Autodesk Inventor part; units mm, degrees
ref_plane "YZ Plane" through (0, 0, 0) normal (1, 0, 0) x (0, 1, 0)
ref_plane "XZ Plane" through (0, 0, 0) normal (0, 1, 0) x (-1, 0, 0)
ref_plane "XY Plane" through (0, 0, 0) normal (0, 0, 1) x (1, 0, 0)
sketch "Boceto1" plane through (0, 0, 0) normal (0, 1, 0) x (-1, 0, 0)
  circle A0 centre (0, 0) radius 10
  circle A1 centre (0, 0) radius 3.5
  dimension "d0" = 20
  dimension "d1" = 7
extrude "Extrusión1" add sketch "Boceto1" along normal blind 4
sketch "Boceto2" plane through (0, 4, 0) normal (0, 1, 0) x (1, 0, 0)
  circle A0 centre (0, 0) radius 8
  circle A1 centre (0, 0) radius 3.5
  circle A2 centre (0, 0) radius 10
  dimension "d4" = 16
extrude "Extrusión2" cut sketch "Boceto2" against normal blind 3 contours A2
sketch "Boceto3" plane through (0, 4, 0) normal (0, 1, 0) x (1, 0, 0)
  circle A0 centre (0, 0) radius 8
  circle A1 centre (0, 0) radius 3.5
  circle A2 centre (0, 0) radius 10
  dimension "d7" = 16
extrude "Extrusión3" add sketch "Boceto3" against normal blind 1 contours A2
fillet "Empalme1" radius 0.5 4 edges at (-8, 1, 0) (-8, 3, 0) (-10, 3, 0) (10, 1, 0)
properties part number "servo pulley"
Read the model definition and answer for the solid it produces. Units are mm, in the model's axes. A direction names the side the tool comes from. Coordinates: 2 decimals unless noted, no trailing zeros. Loops run counter-clockwise (first coordinate to the right, second up) from the corner with the lowest first, then second, coordinate; pieces in that order, holes last.
Q1. Which of the six approach directions +Z, -Z, +X, -X, +Y, -Y give full straight-line access (tool end or side, diameter ignored) to faces 4 (the face through (-4, 0, 0)), 5 (the face through (-2.2, 3, 8.4))?
Q2. Consider probe 1 along Y at (x, z) = (6.25, 7.25); probe 2 along Z at (x, y) = (0, 1.85); probe 3 along Z at (x, y) = (-2, 0.2). Determine where each line is inside the solid, lowest interval first.
Q3. The mould has two halves that part along X. Classify faces 1 (the face through (2.17, 0.25, 9.76)), 2 (the face through (-3.233, 1.972, 1.341)), 3 (the face through (-2.2, 1, 8.4)): +X half, -X half, draft (parallel to the pull), parting line (faces both ways), or undercut.
Q4. The part is cut by section A-A on x = 0. Write down the section's boundary in (y, z).
Q5. The part is cut by section B-B on z = 0. Write down the section's boundary in (x, y), and give its area (3 significant figures).
Results below:
1. face 4: +Z, -Z, +X, -X, -Y
1. face 5: none
2. probe 1: y = 0 to 0.99, 3.01 to 4
2. probe 2: z = -8 to -3.5, 3.5 to 8
2. probe 3: z = -9.8 to -2.87, 2.87 to 9.8
3. face 1: parting line
3. face 2: undercut
3. face 3: draft
4. outline: (0, -10) - (0.5, -10) arc R0.5 ccw to (1, -9.5) - (1, -8.5) arc R0.5 cw to (1.5, -8) - (2.5, -8) arc R0.5 cw to (3, -8.5) - (3, -9.5) arc R0.5 ccw to (3.5, -10) - (4, -10) - (4, -3.5) - (0, -3.5) - close; (0, 3.5) - (4, 3.5) - (4, 10) - (3.5, 10) arc R0.5 ccw to (3, 9.5) - (3, 8.5) arc R0.5 cw to (2.5, 8) - (1.5, 8) arc R0.5 cw to (1, 8.5) - (1, 9.5) arc R0.5 ccw to (0.5, 10) - (0, 10) - close
5. outline: (-10, 0) - (-3.5, 0) - (-3.5, 4) - (-10, 4) - (-10, 3.5) arc R0.5 ccw to (-9.5, 3) - (-8.5, 3) arc R0.5 cw to (-8, 2.5) - (-8, 1.5) arc R0.5 cw to (-8.5, 1) - (-9.5, 1) arc R0.5 ccw to (-10, 0.5) - close; (3.5, 0) - (10, 0) - (10, 0.5) arc R0.5 ccw to (9.5, 1) - (8.5, 1) arc R0.5 cw to (8, 1.5) - (8, 2.5) arc R0.5 cw to (8.5, 3) - (9.5, 3) arc R0.5 ccw to (10, 3.5) - (10, 4) - (3.5, 4) - close
5. area: 44.0 mm2
